Input: dimensioned drawing with shaded views. Units: mm. Origin: part minimum x, y, z. A direction names the side the tool comes from. Round coordinates to 2 decimals unless told otherwise and drop trailing zeros. Loops run counter-clockwise (first coordinate to the right, second up) from the corner with the lowest first, then second, coordinate; pieces in that order, holes last.
Item 1: Section query C-C on z = 6.25. Return loops of the section in (x, y) (1 decimal), then the cut area to 3 significant figures.
Item 2: Access query for the marked faces 1, 2, 3 and 4. Directions: +Z, -Z, +X, -X, +Y, -Y. A direction counts if a zero-diameter tool reaches every point of the face in a straight line with its end or side. Return the directions, or none.
Item 3: Section query A-A on x = 3.75. Return loops of the section in (y, z) (1 decimal).
Item 4: Section query D-D on y = 17. Return loops of the section in (x, z).
Item 5: Ray query, L1, parallel to Y at x = 11.25, z = 2.5; L2, parallel to Z at x = 14.5, y = 15.5; L3, parallel to X at y = 9.5, z = 2.25. Return the intervals inside material, ascending.
Item 6: Section query B-B on y = 13.5. Return loops of the section in (x, z).
Item 7: First-contact query: P1, Ø6, axis at x = 4.5, z = 4.5, coming from the -Y side; P2, Ø2.5, axis at x = 8, z = 2, coming from the -Y side; P3, Ø1, axis at x = 15, z = 12, coming from the -Y side (1 decimal). Flat tips, straight axial feed; report the tip coordinate or a pass-through.
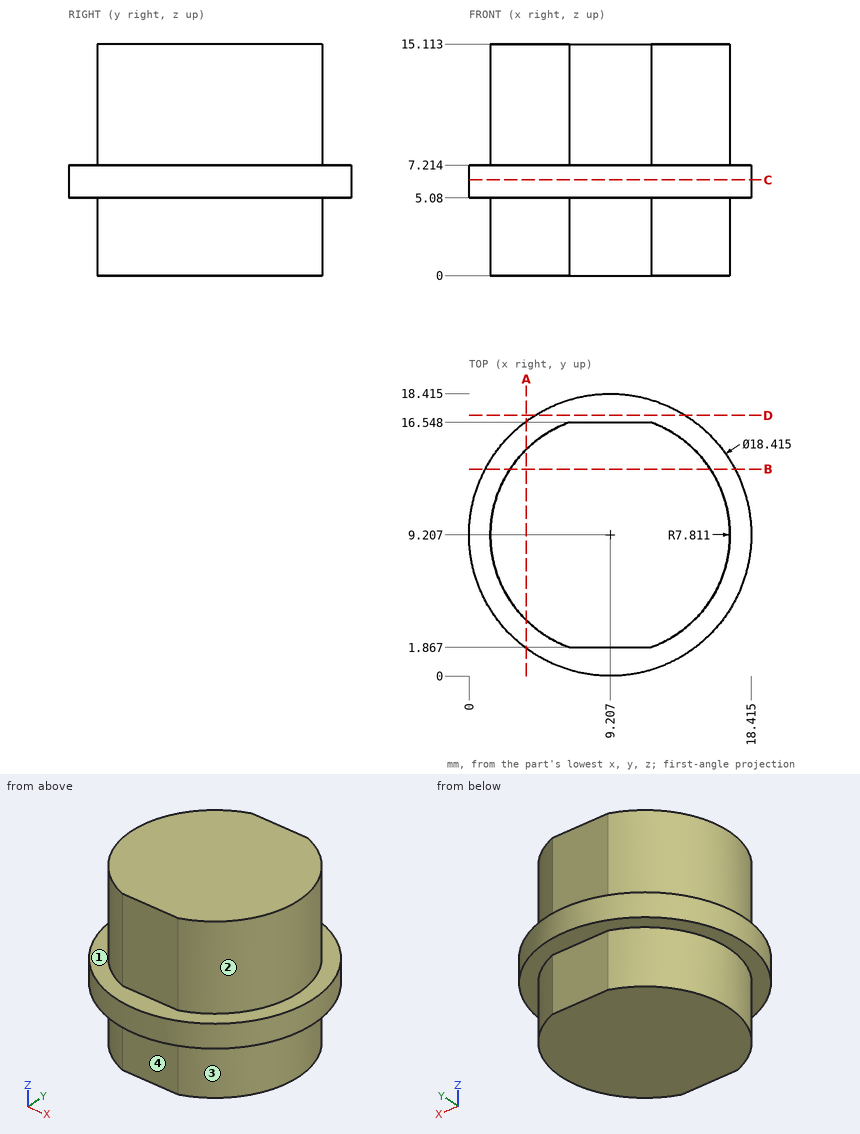
Data:
1. outline: circle Ø18.4 at (9.2, 9.2)
1. area: 266 mm2
2. face 1: +Z
2. face 2: +Z, +X
2. face 3: -Z, +X
2. face 4: -Z, +X, -X, -Y
3. outline: (1.8, 5.1) - (3.6, 5.1) - (3.6, 0) - (14.8, 0) - (14.8, 5.1) - (16.6, 5.1) - (16.6, 7.2) - (14.8, 7.2) - (14.8, 15.1) - (3.6, 15.1) - (3.6, 7.2) - (1.8, 7.2) - close
4. outline: (4.3, 5.08) - (14.11, 5.08) - (14.11, 7.21) - (4.3, 7.21) - close
5. L1: y = 1.87 to 16.55
5. L2: z = 5.08 to 7.21
5. L3: x = 1.4 to 17.01
6. outline: (1.06, 5.08) - (2.68, 5.08) - (2.68, 0) - (15.73, 0) - (15.73, 5.08) - (17.35, 5.08) - (17.35, 7.21) - (15.73, 7.21) - (15.73, 15.11) - (2.68, 15.11) - (2.68, 7.21) - (1.06, 7.21) - close
7. P1: stops at y = 0.17
7. P2: stops at y = 1.87
7. P3: stops at y = 3.5
